from build123d import *

# Parameters (mm, degrees)
F0_R     = 8.8899932806
F0_R_2   = 1.778
F1_DEPTH = 61.722
F2_R     = 1.778
F3_DEPTH = 9.398
F4_SIZE  = 3.81
F5_R     = 6.35
F7_D     = 3.3


with BuildPart() as f1:
    # F0 (on Top) → F1 (new body)
    with BuildSketch(Plane.XY):
        with Locations((-23.340139538, 17.4584258348)):
            Circle(F0_R)
        with Locations((-23.340139538, 17.4584258348)):
            Circle(F0_R_2, mode=Mode.SUBTRACT)
    extrude(amount=F1_DEPTH)

    # F2 (on face) → F3 (join)
    with BuildSketch(Plane.XY.offset(61.722)):
        with BuildLine():
            Line((-15.0224858004, 20.3939921487), (-31.7314702397, 20.3939921487))
            Line((-31.7314702397, 20.3939921487), (-31.7314702397, 14.5228595208))
            ThreePointArc((-31.7314702397, 14.5228595208), (-31.6952463883, 14.4212939558), (-31.6577932757, 14.3201752346))
            Line((-31.6577932757, 14.3201752346), (-15.0224858004, 14.3201752346))
            Line((-15.0224858004, 14.3201752346), (-15.0224858004, 20.3939921487))
        make_face()
        with Locations((-23.340139538, 17.4584258348)):
            Circle(F2_R, mode=Mode.SUBTRACT)
    extrude(amount=F3_DEPTH)

    # F4
    f4_edges = [f1.edges().sort_by_distance(p)[0] for p in [
        (-15.022486, 17.357084, 71.12),
        (-31.73147, 17.458426, 71.12),
    ]]
    chamfer(f4_edges, length=F4_SIZE)

    # F5
    f5_edges = [f1.edges().sort_by_distance(p)[0] for p in [
        (-27.92147, 17.357084, 71.12),
        (-18.832486, 17.357084, 71.12),
        (-15.022486, 17.357084, 67.31),
        (-31.73147, 17.458426, 67.31),
    ]]
    fillet(f5_edges, radius=F5_R)

    # F7 (through all)
    with Locations(Plane.XZ.offset(-14.3201752346)):
        with Locations((-23.3769780201, 66.7147636414)):
            Hole(F7_D / 2)


solid = f1.part
Model file for the job. Use its own axes, mm. A direction names the side the tool comes from. Give positions to 0.01 mm unless a question says otherwise; leave off trailing zeros. Loops run counter-clockwise (first coordinate to the right, second up) from the corner with the lowest first, then second, coordinate; pieces in that order, holes last. Notation, with made-up numbers: (51.5, 71.5) -> (109.5, 71.5) arc R27 ccw to (109.5, 108.5) -> close; hole circle Ø2 at (77.5, 31). An arc over 180 degrees is marked (long way). Use a Markdown table: item, result. Add a question column.
(1) Slice it at D-D on x = -31. List the corners of the cut face in (y, z).
(2) Drop flat-ended pins along their axis: pin 1 Ø3 at (y, z) = (15.5, 30) entering from +X; pin 2 Ø3 at (x, z) = (-26.5, 43) entering from +Y; pin 3 Ø5 at (x, y) = (-17.5, 20) entering from +Z; pin 4 Ø3 at (x, z) = (-23.38, 66.71) entering from -Y. Give the stop position or say it passes through.
(3) Slice it at A-A on x = -27. List the corners of the cut face in (y, z), and give its area (3 significant figures).
(4) Slice it at C-C on y = 23.5. List the corners of the cut face in (x, z), and give its area (3 significant figures).
(5) Mould opens along X. For faces 1 (the flat face through (-31.731, 17, 63)), 2 (the flat face through (-23, 14.32, 64)), 3 (the cylindrical face through (-21.644, 17.992, 35.062)) say: +X half, -X half, draft (parallel to the pull), parting line (faces both ways), or undercut.
(6) Tool access for faces 4 (the flat face through (-15.022, 17, 63)), 5 (the flat face through (-23, 20.394, 64)), 6 (the flat face through (-23, 12, 61.722)), 7 (the cylindrical face through (-27.69, 17.31, 70.65)): list every direction of +Z, -Z, +X, -X, +Y, -Y with a clear straight run to the whole face (end or side of a thin tool).
(7) Wall check: line 1 along X through (y, z) = (17.25, 16); line 2 along X through (y, z) = (16.5, 68); line 3 along Z through (x, y) = (-20.25, 11.5). Give the ranges that are in metal, low to high.
(8) Slice it at B-B on z = 61. List the corners of the cut face in (x, y), and give its area (3 significant figures).
Filled sheet:
| question | item | result |
|---|---|---|
| 1 | outline | (12.95, 0) -> (21.97, 0) -> (21.97, 61.72) -> (20.39, 61.72) -> (20.39, 67.64) -> (14.32, 67.64) -> (14.32, 61.72) -> (12.95, 61.72) -> close |
| 2 | pin 1 | x = -14.46 |
| 2 | pin 2 | y = 26.19 |
| 2 | pin 3 | z = 70.95 |
| 2 | pin 4 | through |
| 3 | outline | (9.36, 0) -> (25.56, 0) -> (25.56, 61.72) -> (20.39, 61.72) -> (20.39, 70.89) -> (14.32, 70.89) -> (14.32, 61.72) -> (9.36, 61.72) -> close |
| 3 | area | 1,060 mm2 |
| 4 | outline | (-29.86, 0) -> (-16.82, 0) -> (-16.82, 61.72) -> (-29.86, 61.72) -> close |
| 4 | area | 805 mm2 |
| 5 | face 1 | -X half |
| 5 | face 2 | draft |
| 5 | face 3 | undercut |
| 6 | face 4 | +Z, +X, +Y, -Y |
| 6 | face 5 | +Z, +X, -X, +Y |
| 6 | face 6 | +Z, +X, -X, -Y |
| 6 | face 7 | +Z, -X, +Y, -Y |
| 7 | line 1 | -32.23 to -25.11, -21.57 to -14.45 |
| 7 | line 2 | -30.79 to -24.84, -21.84 to -15.96 |
| 7 | line 3 | 0 to 61.72 |
| 8 | outline | circle Ø17.78 at (-23.34, 17.46); hole circle Ø3.56 at (-23.34, 17.46) |
| 8 | area | 238 mm2 |
